Build history of the part. All positions in model axes, mm. A direction names the side the tool comes from. Coordinates: 2 decimals unless noted, no trailing zeros. Loops run counter-clockwise (first coordinate to the right, second up) from the corner with the lowest first, then second, coordinate; pieces in that order, holes last. Notation, with made-up numbers: (15, -22.75) - (51, -22.75) arc R12 cw to (51, -9.75) - close; hole circle Ø11 at (-31.75, 41.25). An arc over 180 degrees is marked (long way). One line per item, written item: value.
```python
from build123d import *

# Parameters (mm, degrees)
SKETCH023_W  = 3.3
SKETCH023_H  = 2.2
PAD017_DEPTH = 2.5
PAD018_DEPTH = 5.5
FILLET002_R  = 1.1


with BuildPart() as clone_button_hole:
    # Sketch023 → Pad017 (new body)
    with BuildSketch(Plane.XY):
        Rectangle(SKETCH023_W, SKETCH023_H)
    extrude(amount=PAD017_DEPTH)


with BuildPart() as cut_button_med_final:
    # Sketch024 → Pad018 (new body)
    with BuildSketch(Plane.XY):
        with BuildLine():
            ThreePointArc((4.152027, 3), (0, 3.158098), (-4.152027, 3))
            ThreePointArc((-4.152027, 3), (-5.105717, 2.54284), (-5.499998, 1.561482))
            ThreePointArc((-5.499998, 1.561482), (-5.508705, 0), (-5.5, -1.561483))
            ThreePointArc((-5.5, -1.561483), (-5.105718, -2.542841), (-4.152027, -3))
            ThreePointArc((-4.152027, -3), (0, -3.158098), (4.152027, -3))
            ThreePointArc((4.152027, -3), (5.105718, -2.542841), (5.5, -1.561483))
            ThreePointArc((5.5, -1.561483), (5.508705, 0), (5.499998, 1.561482))
            ThreePointArc((5.499998, 1.561482), (5.105717, 2.54284), (4.152027, 3))
        make_face()
    extrude(amount=PAD018_DEPTH)

    # Fillet002
    fillet002_edges = [cut_button_med_final.edges().sort_by_distance(p)[0] for p in [
        (0, 3.158098, 5.5),
        (-5.105717, 2.54284, 5.5),
        (-5.508705, 0, 5.5),
        (-5.105718, -2.542841, 5.5),
        (0, -3.158098, 5.5),
        (5.105718, -2.542841, 5.5),
        (5.508705, 0, 5.5),
        (5.105717, 2.54284, 5.5),
    ]]
    fillet(fillet002_edges, radius=FILLET002_R)

    # Cut005: cut Clone (button hole)
    add(clone_button_hole.part, mode=Mode.SUBTRACT)


solid = cut_button_med_final.part
```
Item 1: Tool access for faces 5 (the face through (0, 1.1, 1)), 6 (the face through (-0.1, -1.4, 0)): list every direction of +Z, -Z, +X, -X, +Y, -Y with a clear straight run to the whole face (end or side of a thin tool).
Check result:
face 5: -Z
face 6: -Z, +X, -X, +Y, -Y
Item 2: Cut at B-B, the plane z = 4.05. Write the cut outline in (x, y).
Check result:
outline: (-5.5, -1.56) arc R1.46 ccw to (-4.15, -3) arc R54.6 ccw to (4.15, -3) arc R1.46 ccw to (5.5, -1.56) arc R140.04 ccw to (5.5, 1.56) arc R1.46 ccw to (4.15, 3) arc R54.6 ccw to (-4.15, 3) arc R1.46 ccw to (-5.5, 1.56) arc R140.04 ccw to start
Item 3: Drop flat-ended pins along their axis: P1, Ø1, axis at x = 2, z = 2.5, coming from the +Y side; P2, Ø2, axis at x = -4.5, y = -1.5, coming from the -Z side; P3, Ø0.7, axis at x = -0.5, y = 0, coming from the -Z side. Give the stop position or say it passes through.
Check result:
P1: stops at y = 3.14
P2: stops at z = 0
P3: stops at z = 2.5
Item 4: Pull direction Y, two halves, no side cores. Call faces 1 (the face through (-5.1, 2.55, 2.17)), 2 (the face through (-1.65, 0, 1)), 3 (the face through (1.65, 0, 1)), 4 (the face through (5.1, -2.55, 2.17)): released by +Y, released by -Y, zero draft, split by the parting line, or undercut.
Check result:
face 1: released by +Y
face 2: undercut
face 3: undercut
face 4: released by -Y
Item 5: Probe probe 1 along X at (y, z) = (0.5, 2.3); probe 2 along X at (y, z) = (1.25, 0.75); probe 3 along Z at (x, y) = (0.75, 0). List the from-to ranges inside material, lowest first. Write a range as from..to.
Check result:
probe 1: x = -5.51..-1.65, 1.65..5.51
probe 2: x = -5.5..5.5
probe 3: z = 2.5..5.5
Item 6: Cut at A-A, the plane z = 0.75. Write the cut outline in (x, y), then the cut area to 3 significant figures.
Check result:
outline: (-5.5, -1.56) arc R1.46 ccw to (-4.15, -3) arc R54.6 ccw to (4.15, -3) arc R1.46 ccw to (5.5, -1.56) arc R140.04 ccw to (5.5, 1.56) arc R1.46 ccw to (4.15, 3) arc R54.6 ccw to (-4.15, 3) arc R1.46 ccw to (-5.5, 1.56) arc R140.04 ccw to start; hole (-1.65, -1.1) - (1.65, -1.1) - (1.65, 1.1) - (-1.65, 1.1) - close
area: 58.7 mm^2
